from build123d import *

# Parameters (mm, degrees)
F0_R     = 36
F0_R_2   = 27
F1_DEPTH = 40
F2_R     = 29.975
F3_DEPTH = 33
F4_SIZE  = 5
F5_SIZE  = 1


with BuildPart() as f1:
    # F0 (on Top) → F1 (new body)
    with BuildSketch(Plane.XY):
        Circle(F0_R)
        Circle(F0_R_2, mode=Mode.SUBTRACT)
    extrude(amount=F1_DEPTH)

    # F2 (on face) → F3 (cut)
    with BuildSketch(Plane.XY.offset(40)):
        Circle(F2_R)
    extrude(amount=-F3_DEPTH, mode=Mode.SUBTRACT)

    # F4
    f4_edges = [f1.edges().sort_by_distance(p)[0] for p in [
        (-27, 0, 0),
    ]]
    chamfer(f4_edges, length=F4_SIZE)

    # F5
    f5_edges = [f1.edges().sort_by_distance(p)[0] for p in [
        (-36, 0, 0),
        (-36, 0, 40),
        (-29.975, 0, 40),
    ]]
    chamfer(f5_edges, length=F5_SIZE)


solid = f1.part
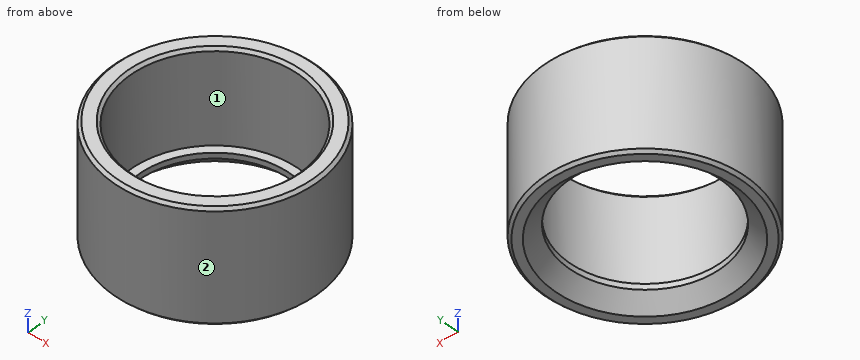
Design review of the part built by this model. Coordinates are the model's own, in mm. Face numbers are marked on the shaded views. Give positions to 0.01 mm unless a question says otherwise; leave off trailing zeros. Loops run counter-clockwise (first coordinate to the right, second up) from the corner with the lowest first, then second, coordinate; pieces in that order, holes last. Notation, with made-up numbers: M 59.5,69.25 L 108.5,69.25 A30 ccw 108.5,105.25 Z; hole C 67.5,-17.5 d8. An arc over 180 degrees is marked long. One line per question, with ' | ' between items. Start each with the question number.
1. Add section C-C (z = 12). Write out the cut boundary in (x, y) (3 decimals).
2. Insertion check: P1, Ø1.5, axis at y = 28, z = 27.5, coming from the +X side; P2, Ø1, axis at y = -14.5, z = 15.5, coming from the -X side; P3, Ø3, axis at y = 7.5, z = 32, coming from the +X side. Each pin has a flat end and moves straight along its axis. Give the tip position at first contact, or say it passes through.
3. Add section D-D (z = 4). Write out the cut boundary in (x, y).
4. To check wall thickness, follow L1, parallel to X at y = 1, z = 20.5; L2, parallel to Y at x = 0, z = 6.6; L3, parallel to Y at x = 6, z = 20.5. State the ranges of each line that lie inside material, in increasing order.
5. The part is to be moulded in two halves that separate along Y. For the marked faces 1 and 2, say which applies: released by +Y, released by -Y, zero draft, split by the parting line, or undercut.
6. Add section A-A (x = 0). Write out the cut boundary in (y, z) (3 decimals), plus the area to 3 significant figures.
Worked out:
1) outline: C 0,0 d72; hole C 0,0 d59.95
2) P1: stops at x = 23.53 | P2: stops at x = -33.17 | P3: stops at x = 35.5
3) outline: C 0,0 d72; hole C 0,0 d56
4) L1: x = -35.99 to -29.96, 29.96 to 35.99 | L2: y = -36 to -27, 27 to 36 | L3: y = -35.5 to -29.37, 29.37 to 35.5
5) face 1: undercut | face 2: split by the parting line
6) outline: M -36,1 L -35,0 L -32,0 L -27,5 L -27,7 L -29.975,7 L -29.975,39 L -30.975,40 L -35,40 L -36,39 Z; M 27,5 L 32,0 L 35,0 L 36,1 L 36,39 L 35,40 L 30.975,40 L 29.975,39 L 29.975,7 L 27,7 Z | area: 496 mm²
